Read the model definition and answer for the solid it produces. Units are mm, in the model's axes. A direction names the side the tool comes from. Round coordinates to 2 decimals unless told otherwise and drop trailing zeros. Write each loop counter-clockwise with the first axis right and the second up, starting at its lowest first coordinate (ties: lowest second). Pieces come first, ordered by that corner, then holes. Notation, with made-up numbers: (28.5, -38.75) -> (52.5, -38.75) arc R19 cw to (52.5, -28.75) -> close; hole circle Ø3 at (16.5, -2.75). An arc over 180 degrees is marked (long way). Return JSON: item names as keys, results as strings. Group by question number.
(1) A cutting plane is placed at A-A on x = 6. Give the vertices of the cut face in (y, z), then the cut area to 3 significant figures.
(2) For faces 1 (the flat face through (18, 0, 0)), 2 (the flat face through (-1, -0.996, 0)), determine the directions among +Z, -Z, +X, -X, +Y, -Y from which every point of the face is accessible in a straight line to the end or side of a thin tool.
(3) Straight lines are drawn through the part: line 1 (X direction, y = -0.65, z = 0.2); line 2 (Y direction, x = -0.75, z = -1.05); line 3 (Y direction, x = 7.5, z = 0.95). For each, find the intervals that lie inside material, in ascending order.
(4) The mould has two halves that part along Z. Classify faces 3 (the flat face through (-1.41, -0.5, -0.86)), 4 (the flat face through (0, 2, 0)), 5 (the cylindrical face through (8.88, -1.5, -0.07)): released by +Z, released by -Z, zero draft, split by the parting line, or undercut.
(5) Given pin 1 (1.3 mm diameter, centred on x = -1.5, z = 0, fed in from +Y), flat-ended and moving along its own axis, determine where the tip first touches the part or whether it passes through.
Autodesk Inventor part; units mm, degrees
ref_plane "YZ Plane" through (0, 0, 0) normal (1, 0, 0) x (0, 1, 0)
ref_plane "XZ Plane" through (0, 0, 0) normal (0, 1, 0) x (-1, 0, 0)
ref_plane "XY Plane" through (0, 0, 0) normal (0, 0, 1) x (1, 0, 0)
sketch "スケッチ1" plane through (0, 0, 0) normal (0, 0, 1) x (1, 0, 0)
  line L0 (0, 0) -> (18, 0)
  line L1 (18, 0) -> (18, 1.5)
  line L2 (18, 1.5) -> (0, 1.5)
  line L3 (0, 1.5) -> (0, 0)
  line L4 (0, 0) -> (0, 2.75)
  line L5 (0, 0) -> (-2, 0)
  line L6 (-2, 0) -> (0, 0)
  line L7 (-2, 0) -> (-2, 1.15)
  arc A0 (0, 2.75) -> (-2, 1.15) centre (-0.0403, 0.7504) ccw
  dimension "d0" = 1.5
  dimension "d1" = 18
  dimension "d3" = 2
  dimension "d4" = 2.75
  dimension "d5" = 1.15
  dimension "d6" = 2
revolve "回転1" add sketch "スケッチ1" angle 360 about axis through (-2, 0, 0) along (1, 0, 0)
thread "ねじ1"
sketch "スケッチ2" plane through (-2, 0, 0) normal (-1, 0, 0) x (0, 0, 1)
  circle A0 centre (0, 0) radius 1.15
  line L0 (-0.575, 0.9959) -> (0.575, 0.9959)
  line L1 (0.575, 0.9959) -> (1.15, 0)
  line L2 (1.15, 0) -> (0.575, -0.9959)
  line L3 (0.575, -0.9959) -> (-0.575, -0.9959)
  line L4 (-0.575, -0.9959) -> (-1.15, 0)
  line L5 (-1.15, 0) -> (-0.575, 0.9959)
  dimension "d10" = 1.15
  dimension "d11" = 1.9919
extrude "押し出し1" cut sketch "スケッチ2" against normal blind 1.4 contours L2 L3 L4 L5 L0 L1
fillet "フィレット1" radius 0.2 6 edges at (-0.6, 0.9959, 0) (-0.6, 0.498, 0.8625) (-0.6, 0.498, -0.8625) (-0.6, -0.498, -0.8625) (-0.6, -0.9959, 0) (-0.6, -0.498, 0.8625)
fillet "フィレット2" radius 0.1 1 edges at (0, -1.5, 0)
fillet "フィレット3" radius 0.1 1 edges at (18, -1.5, 0)
properties part number "ネジボタンM3L18" material "鋼"
Checks:
{
 "1": {"outline": "circle Ø3 at (0, 0)", "area": "7.07 mm^2"},
 "2": {"face 1": "+Z, -Z, +X, +Y, -Y", "face 2": "-X"},
 "3": {"line 1": "x = -0.6 to 18", "line 2": "y = -2.4 to -0.16, 0.16 to 2.4", "line 3": "y = -1.16 to 1.16"},
 "4": {"face 3": "undercut", "face 4": "zero draft", "face 5": "split by the parting line"},
 "5": {"pin 1": "stops at y = 2.58"}
}
